Build history of the part. All positions in model axes, mm. Face numbers are marked on the shaded views. Give positions to 0.01 mm unless a question says otherwise; leave off trailing zeros. Write each loop counter-clockwise with the first axis right and the second up, starting at its lowest first coordinate (ties: lowest second). Pieces come first, ordered by that corner, then holes. Notation, with made-up numbers: (33.25, -38.5) - (46.25, -38.5) arc R35 cw to (46.25, -5.5) - close; hole circle Ø7 at (-37.5, 48.5). An arc over 180 degrees is marked (long way). Use one line per item in the form item = value. Start each with the question number.
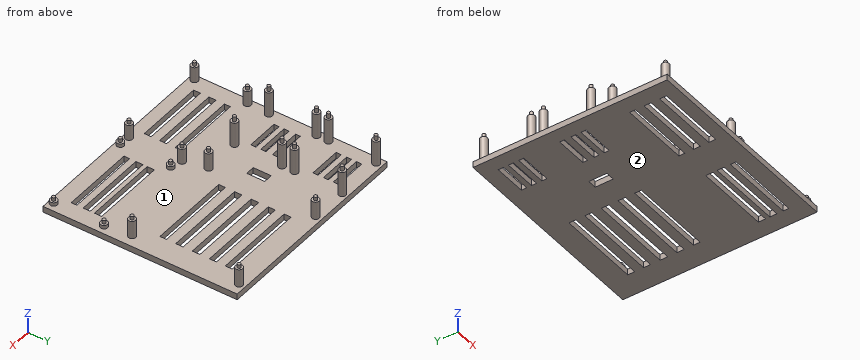
from build123d import *

# Parameters (mm, degrees)
SKETCH1_R            = 3
SKETCH1_W            = 57.32549759
SKETCH1_H            = 5.688771297
SKETCH1_H_2          = 5.842521873
SKETCH1_H_3          = 4.92001842
SKETCH1_W_2          = 26.922884564
SKETCH1_H_4          = 4.277382824
SKETCH1_W_3          = 61.334124095
SKETCH1_H_5          = 4.704767614
SKETCH1_H_6          = 5.974747368
SKETCH1_W_4          = 68.406104656
SKETCH1_H_7          = 5.494466237
SKETCH1_H_8          = 4.269416466
SKETCH1_H_9          = 3.943377121
SKETCH1_W_5          = 7.5
SKETCH1_H_10         = 15
SKETCH1_H_11         = 4.248368433
SKETCH1_H_12         = 4.139435909
SKETCH1_H_13         = 4.46623348
SKETCH1_H_14         = 6.107283804
SKETCH1_H_15         = 6.318636173
SKETCH1_H_16         = 5.769189549
SKETCH1_H_17         = 5.76918955
BOSS_EXTRUDE3_DEPTH  = 5
SKETCH1_6_R          = 3
BOSS_EXTRUDE4_DEPTH  = 26
SKETCH1_8_R          = 3
BOSS_EXTRUDE5_DEPTH  = 18
SKETCH1_10_R         = 3
BOSS_EXTRUDE6_DEPTH  = 8
SKETCH1_11_R         = 3
BOSS_EXTRUDE7_DEPTH  = 20
SKETCH1_12_R         = 1.4
BOSS_EXTRUDE8_DEPTH  = 30
SKETCH1_13_R         = 1.4
BOSS_EXTRUDE9_DEPTH  = 21
SKETCH1_15_R         = 1.4
BOSS_EXTRUDE10_DEPTH = 11
SKETCH1_16_R         = 1.4
BOSS_EXTRUDE11_DEPTH = 23


with BuildPart() as part:
    # Sketch1 → Boss-Extrude3 (new body)
    with BuildSketch(Plane.XY):
        Polygon((-20.116410516, 63.581349206), (-73.848571429, 63.581349206), (-73.848571429, -97.918650794), (100.383589484, -97.918650794), (100.383589484, -60.85880545), (100.383589484, -37.85880545), (100.383589484, 63.581349206), (2.883589484, 63.581349206), align=None)
        with Locations((-69.478571429, -93.418650794)):
            Circle(SKETCH1_R, mode=Mode.SUBTRACT)
        with Locations((-31.584870297, -84.690322091)):
            Rectangle(SKETCH1_W, SKETCH1_H, mode=Mode.SUBTRACT)
        with Locations((-31.584870297, -71.852149028)):
            Rectangle(SKETCH1_W, SKETCH1_H_2, mode=Mode.SUBTRACT)
        with Locations((-31.584870297, -59.398352403)):
            Rectangle(SKETCH1_W, SKETCH1_H_3, mode=Mode.SUBTRACT)
        with Locations((6.601428571, -93.418650794)):
            Circle(SKETCH1_R, mode=Mode.SUBTRACT)
        with Locations((16.141428571, -93.878650794)):
            Circle(SKETCH1_R, mode=Mode.SUBTRACT)
        with Locations((-69.523792896, -49.418650794)):
            Circle(SKETCH1_R, mode=Mode.SUBTRACT)
        with Locations((-68.788571429, -31.080828543)):
            Circle(SKETCH1_R, mode=Mode.SUBTRACT)
        with Locations((-28.788571429, -31.080828543)):
            Circle(SKETCH1_R, mode=Mode.SUBTRACT)
        with Locations((-48.537699589, -19.846770176)):
            Rectangle(SKETCH1_W_2, SKETCH1_H_4, mode=Mode.SUBTRACT)
        with Locations((6.556207104, -49.418674032)):
            Circle(SKETCH1_R, mode=Mode.SUBTRACT)
        with Locations((16.141428571, -51.968650794)):
            Circle(SKETCH1_R, mode=Mode.SUBTRACT)
        with Locations((2.071428571, -30.498650794)):
            Circle(SKETCH1_R, mode=Mode.SUBTRACT)
        with Locations((55.384741084, -82.337938284)):
            Rectangle(SKETCH1_W_3, SKETCH1_H_5, mode=Mode.SUBTRACT)
        with Locations((55.384741084, -71.852149028)):
            Rectangle(SKETCH1_W_3, SKETCH1_H_2, mode=Mode.SUBTRACT)
        with Locations((55.384741084, -62.385726087)):
            Rectangle(SKETCH1_W_3, SKETCH1_H_6, mode=Mode.SUBTRACT)
        with Locations((93.611428571, -93.878650794)):
            Circle(SKETCH1_R, mode=Mode.SUBTRACT)
        with Locations((46.379204663, -12.094485759)):
            Rectangle(SKETCH1_W_4, SKETCH1_H_7, mode=Mode.SUBTRACT)
        with Locations((93.611428571, -51.968650794)):
            Circle(SKETCH1_R, mode=Mode.SUBTRACT)
        with Locations((91.071428571, -30.498650794)):
            Circle(SKETCH1_R, mode=Mode.SUBTRACT)
        with Locations((-68.788571429, 8.581349206)):
            Circle(SKETCH1_R, mode=Mode.SUBTRACT)
        with Locations((-48.537699589, -11.481960873)):
            Rectangle(SKETCH1_W_2, SKETCH1_H_8, mode=Mode.SUBTRACT)
        with Locations((-48.537699589, -1.971688561)):
            Rectangle(SKETCH1_W_2, SKETCH1_H_9, mode=Mode.SUBTRACT)
        with Locations((-28.788571429, 8.581349206)):
            Circle(SKETCH1_R, mode=Mode.SUBTRACT)
        with Locations((-68.788571429, 18.581349206)):
            Circle(SKETCH1_R, mode=Mode.SUBTRACT)
        with Locations((-28.788571429, 18.91917133)):
            Circle(SKETCH1_R, mode=Mode.SUBTRACT)
        with Locations((-12.366410516, 1.081349206)):
            Rectangle(SKETCH1_W_5, SKETCH1_H_10, mode=Mode.SUBTRACT)
        with Locations((-48.537699589, 31.881415248)):
            Rectangle(SKETCH1_W_2, SKETCH1_H_11, mode=Mode.SUBTRACT)
        with Locations((-48.537699589, 40.541550899)):
            Rectangle(SKETCH1_W_2, SKETCH1_H_12, mode=Mode.SUBTRACT)
        with Locations((-48.537699589, 48.874888978)):
            Rectangle(SKETCH1_W_2, SKETCH1_H_13, mode=Mode.SUBTRACT)
        with Locations((-68.248571429, 58.581349206)):
            Circle(SKETCH1_R, mode=Mode.SUBTRACT)
        with Locations((-28.248571429, 58.91917133)):
            Circle(SKETCH1_R, mode=Mode.SUBTRACT)
        with Locations((2.071428571, 58.501349206)):
            Circle(SKETCH1_R, mode=Mode.SUBTRACT)
        with Locations((46.379204663, 1.398641994)):
            Rectangle(SKETCH1_W_4, SKETCH1_H_14, mode=Mode.SUBTRACT)
        with Locations((46.379204663, 15.240483772)):
            Rectangle(SKETCH1_W_4, SKETCH1_H_15, mode=Mode.SUBTRACT)
        with Locations((46.379204663, 29.251372679)):
            Rectangle(SKETCH1_W_4, SKETCH1_H_16, mode=Mode.SUBTRACT)
        with Locations((46.379204663, 42.438091648)):
            Rectangle(SKETCH1_W_4, SKETCH1_H_17, mode=Mode.SUBTRACT)
        with Locations((91.071428571, 58.501349206)):
            Circle(SKETCH1_R, mode=Mode.SUBTRACT)
    extrude(amount=BOSS_EXTRUDE3_DEPTH)

    # Sketch1_6 → Boss-Extrude4 (add)
    with BuildSketch(Plane.XY):
        with Locations(Location((-28.788571429, -31.080828543, 0), (0, 0, 180))):
            Circle(SKETCH1_6_R)
        with Locations(Location((-68.788571429, -31.080828543, 0), (0, 0, 180))):
            Circle(SKETCH1_6_R)
        with Locations(Location((-68.788571429, 8.581349206, 0), (0, 0, 180))):
            Circle(SKETCH1_6_R)
        with Locations(Location((-28.788571429, 8.581349206, 0), (0, 0, 180))):
            Circle(SKETCH1_6_R)
        with Locations(Location((-28.788571429, 18.91917133, 0), (0, 0, 180))):
            Circle(SKETCH1_6_R)
        with Locations(Location((-68.788571429, 18.581349206, 0), (0, 0, 180))):
            Circle(SKETCH1_6_R)
        with Locations(Location((-68.248571429, 58.581349206, 0), (0, 0, 180))):
            Circle(SKETCH1_6_R)
        with Locations(Location((-28.248571429, 58.91917133, 0), (0, 0, 180))):
            Circle(SKETCH1_6_R)
    extrude(amount=BOSS_EXTRUDE4_DEPTH)

    # Sketch1_8 → Boss-Extrude5 (add)
    with BuildSketch(Plane.XY):
        with Locations((6.601428571, -93.418650794)):
            Circle(SKETCH1_8_R)
        with Locations((6.556207104, -49.418674032)):
            Circle(SKETCH1_8_R)
        with Locations((-69.523792896, -49.418650794)):
            Circle(SKETCH1_8_R)
        with Locations((-69.478571429, -93.418650794)):
            Circle(SKETCH1_8_R)
    extrude(amount=BOSS_EXTRUDE5_DEPTH)

    # Sketch1_10 → Boss-Extrude6 (add)
    with BuildSketch(Plane.XY):
        with Locations((93.611428571, -93.878650794)):
            Circle(SKETCH1_10_R)
        with Locations((93.611428571, -51.968650794)):
            Circle(SKETCH1_10_R)
        with Locations((16.141428571, -51.968650794)):
            Circle(SKETCH1_10_R)
        with Locations((16.141428571, -93.878650794)):
            Circle(SKETCH1_10_R)
    extrude(amount=BOSS_EXTRUDE6_DEPTH)

    # Sketch1_11 → Boss-Extrude7 (add)
    with BuildSketch(Plane.XY):
        with Locations((91.071428571, 58.501349206)):
            Circle(SKETCH1_11_R)
        with Locations((2.071428571, 58.501349206)):
            Circle(SKETCH1_11_R)
        with Locations((2.071428571, -30.498650794)):
            Circle(SKETCH1_11_R)
        with Locations((91.071428571, -30.498650794)):
            Circle(SKETCH1_11_R)
    extrude(amount=BOSS_EXTRUDE7_DEPTH)

    # Sketch1_12 → Boss-Extrude8 (add)
    with BuildSketch(Plane.XY):
        with Locations((-28.788571429, -31.080828543)):
            Circle(SKETCH1_12_R)
        with Locations((-68.788571429, -31.080828543)):
            Circle(SKETCH1_12_R)
        with Locations((-68.788571429, 8.581349206)):
            Circle(SKETCH1_12_R)
        with Locations((-68.788571429, 18.581349206)):
            Circle(SKETCH1_12_R)
        with Locations((-28.788571429, 18.91917133)):
            Circle(SKETCH1_12_R)
        with Locations((-68.248571429, 58.581349206)):
            Circle(SKETCH1_12_R)
        with Locations((-28.248571429, 58.91917133)):
            Circle(SKETCH1_12_R)
        with Locations((-28.788571429, 8.581349206)):
            Circle(SKETCH1_12_R)
    extrude(amount=BOSS_EXTRUDE8_DEPTH)

    # Sketch1_13 → Boss-Extrude9 (add)
    with BuildSketch(Plane.XY):
        with Locations(Location((-69.478571429, -93.418650794, 0), (0, 0, 180))):
            Circle(SKETCH1_13_R)
        with Locations(Location((6.601428571, -93.418650794, 0), (0, 0, 180))):
            Circle(SKETCH1_13_R)
        with Locations(Location((-69.523792896, -49.418650794, 0), (0, 0, 180))):
            Circle(SKETCH1_13_R)
        with Locations(Location((6.556207104, -49.418674032, 0), (0, 0, 180))):
            Circle(SKETCH1_13_R)
    extrude(amount=BOSS_EXTRUDE9_DEPTH)

    # Sketch1_15 → Boss-Extrude10 (add)
    with BuildSketch(Plane.XY):
        with Locations((16.141428571, -93.878650794)):
            Circle(SKETCH1_15_R)
        with Locations((93.611428571, -93.878650794)):
            Circle(SKETCH1_15_R)
        with Locations((93.611428571, -51.968650794)):
            Circle(SKETCH1_15_R)
        with Locations((16.141428571, -51.968650794)):
            Circle(SKETCH1_15_R)
    extrude(amount=BOSS_EXTRUDE10_DEPTH)

    # Sketch1_16 → Boss-Extrude11 (add)
    with BuildSketch(Plane.XY):
        with Locations((91.071428571, 58.501349206)):
            Circle(SKETCH1_16_R)
        with Locations((91.071428571, -30.498650794)):
            Circle(SKETCH1_16_R)
        with Locations((2.071428571, -30.498650794)):
            Circle(SKETCH1_16_R)
        with Locations((2.071428571, 58.501349206)):
            Circle(SKETCH1_16_R)
    extrude(amount=BOSS_EXTRUDE11_DEPTH)


solid = part.part
(1) Cut at B-B, the plane y = 53.5. Give the cut face in (x, z).
(2) Cut at A-A, the plane z = 15. State how many separate pieces and enclosed holes the cut face has, then the cut area to 3 significant figures.
(3) Wall check: line 1 (X direction, y = -71.5, z = 3.25); line 2 (Y direction, x = 86, z = 3.5); line 3 (X direction, y = 9, z = 22.25). Give the ranges that are in metal, low to high. Write a range as from..to.
(4) Two-plate mould, pull along X, no slides. Class the marked faces 1 and 2: +X half, -X half, draft (parallel to the pull), parting line (faces both ways), or undercut.
(5) Pin check, flat tips, straight feed: pin 1 Ø1.4 at (x, y) = (92, -30.5) entering from +Z; pin 2 Ø1.5 at (x, y) = (69, -29) entering from +Z; pin 3 Ø0.8 at (x, y) = (16, -51.5) entering from +Z. Stop position of each tip, or through.
Solution:
q1.outline = (-73.85, 0) - (100.38, 0) - (100.38, 5) - (-73.85, 5) - close
q2.separate_pieces = 16
q2.enclosed_holes = 0
q2.area = 452 mm2
q3.line_1 = -73.85..-60.25, -2.92..24.72, 86.05..100.38
q3.line_2 = -97.92..-84.69, -79.99..-74.77, -68.93..-65.37, -59.4..63.58
q3.line_3 = -71.76..-65.82, -31.76..-25.82
q4.face_1 = undercut
q4.face_2 = draft
q5.pin_1 = 23
q5.pin_2 = 5
q5.pin_3 = 11
